```python
from build123d import *

# Parameters (mm, degrees)
BOSS_EXTRU_1_DEPTH      = 6.35
ESQUISSE4_R             = 12.5
BOSS_EXTRU_2_DEPTH      = 6.35
ENL_V_MAT_EXTRU_1_REACH = 85.387
ESQUISSE3_R             = 1.5
ENL_V_MAT_EXTRU_2_DEPTH = 6.35
CONG_1_R                = 4


with BuildPart() as part:
    # Esquisse1 → Boss.-Extru.1 (new body)
    with BuildSketch(Plane.XY):
        with BuildLine():
            Line((0, 6), (76.2, 6))
            ThreePointArc((76.2, 6), (82.2, 0), (76.2, -6))
            Line((76.2, -6), (0, -6))
            ThreePointArc((0, -6), (-6, 0), (0, 6))
        make_face()
    extrude(amount=BOSS_EXTRU_1_DEPTH)

    # Esquisse4 → Boss.-Extru.2 (add)
    with BuildSketch(Plane.XY.offset(6.35)):
        Circle(ESQUISSE4_R)
    extrude(amount=-BOSS_EXTRU_2_DEPTH)

    # Esquisse2 → Enlèv. mat.-Extru.1 (cut, up to next)
    with BuildSketch(Plane.XY.offset(6.35), mode=Mode.PRIVATE) as enl_v_mat_extru_1_sk1:
        with BuildLine():
            Line((-2.886173938, -2.275), (2.886173938, -2.275))
            ThreePointArc((2.886173938, -2.275), (0, 3.675), (-2.886173938, -2.275))
        make_face()
    enl_v_mat_extru_1_tool1 = extrude(enl_v_mat_extru_1_sk1.sketch, amount=-ENL_V_MAT_EXTRU_1_REACH, mode=Mode.PRIVATE) & part.part
    add(enl_v_mat_extru_1_tool1.solids().sort_by_distance((0, 0.435587, 6.35))[0], mode=Mode.SUBTRACT)

    # Esquisse3 → Enlèv. mat.-Extru.2 (cut)
    with BuildSketch(Plane.XY.offset(6.35)):
        with Locations((76.2, 0)):
            Circle(ESQUISSE3_R)
    extrude(amount=-ENL_V_MAT_EXTRU_2_DEPTH, mode=Mode.SUBTRACT)

    # Congé1
    cong_1_edges = [part.edges().sort_by_distance(p)[0] for p in [
        (10.9658561, -6, 3.175),
        (10.9658561, 6, 3.175),
    ]]
    fillet(cong_1_edges, radius=CONG_1_R)


solid = part.part
```
Here's how the part is built. I have some questions about the finished solid (model axes, mm). A direction names the side the tool comes from. Give positions to 0.01 mm unless a question says otherwise; leave off trailing zeros. Write each loop counter-clockwise with the first axis right and the second up, starting at its lowest first coordinate (ties: lowest second). Pieces come first, ordered by that corner, then holes. Notation, with made-up numbers: M -28,64.25 L 0,64.25 A12 cw 0,77.25 Z; hole C -18,61.25 d5. An arc over 180 degrees is marked long. Put each result on its own line as item: value. Start each with the question number.
Item 1: Thinking about a two-plate mould opening in X: for faces 3 (the cylindrical face through (11.326, 6.427, 3.219)), 4 (the flat face through (0, -2.275, 3)), 5 (the flat face through (45, -6, 3)), which applies, +X half, -X half, draft (parallel to the pull), parting line (faces both ways), or undercut?
Item 2: I need wall thicknesses on L1, parallel to Y at x = 76.2, z = 1.5; L2, parallel to Y at x = -1, z = 2.5 (3 decimals); L3, parallel to Y at x = 73.5, z = 5.5. Which ranges of each line are inside material? Lowest first, please. Write a range as from..to.
Item 3: If we section it at A-A, the plane y = 0: Write out the boundary of the cut face in (x, z) (3 decimals), then the cut area to 3 significant figures.
Item 4: If we section it at C-C, the plane x = 0: Write out the boundary of the cut face in (y, z) (3 decimals), then the cut area to 3 significant figures.
Item 5: If we section it at D-D, the plane x = 50: Write out the boundary of the cut face in (y, z), then the cut area to 3 significant figures.
Item 6: On a 3-axis mill with a long thin cutter (end or side, diameter ignored), from which of +Z, -Z, +X, -X, +Y, -Y can I reach the whole of each face in a straight line? I mean faces 1 (the flat face through (44, 6, 3)), 2 (the flat face through (36, 0, 0)). Say none if no direction works.
Item 7: If we section it at B-B, the plane z = 5.25: Write out the boundary of the cut face in (x, y) (3 decimals).
Item 8: Will these pins go through, and if not, where does the flat tip stop? pin 1 (1.5 mm diameter, centred on y = -6.5, z = 2.5, fed in from -X); pin 2 (1.5 mm diameter, centred on x = 64, z = 4.5, fed in from -Y).
Values:
1. face 3: +X half
1. face 4: undercut
1. face 5: draft
2. L1: -6..-1.5, 1.5..6
2. L2: -12.46..-2.275, 3.536..12.46
2. L3: -6..6
3. outline: M -12.5,0 L -3.675,0 L -3.675,6.35 L -12.5,6.35 Z; M 3.675,0 L 74.7,0 L 74.7,6.35 L 3.675,6.35 Z; M 77.7,0 L 82.2,0 L 82.2,6.35 L 77.7,6.35 Z
3. area: 536 mm²
4. outline: M -12.5,0 L -2.275,0 L -2.275,6.35 L -12.5,6.35 Z; M 3.675,0 L 12.5,0 L 12.5,6.35 L 3.675,6.35 Z
4. area: 121 mm²
5. outline: M -6,0 L 6,0 L 6,6.35 L -6,6.35 Z
5. area: 76.2 mm²
6. face 1: +Z, -Z, +X, +Y
6. face 2: -Z, +X, -X, +Y, -Y
7. outline: M 9.943,-7.576 A4 cw 13.124,-6 L 76.2,-6 A6 ccw 76.2,6 L 13.124,6 A4 cw 9.943,7.576 A12.5 ccw long Z; hole M -2.886,-2.275 L 2.886,-2.275 A3.675 ccw long Z; hole C 76.2,0 d3
8. pin 1: x = -11.1
8. pin 2: y = -6
